Design review of the part built by this model. Coordinates are the model's own, in mm. Face numbers are marked on the shaded views. Round coordinates to 2 decimals unless told otherwise and drop trailing zeros. Order: outer loops, then holes, each group sorted by start corner. A loop starts at its lowest first (then second) coordinate and runs counter-clockwise, first axis right, second up. Notation, with made-up numbers: (14.5, 18.25) - (25.5, 18.25) arc R34 cw to (25.5, 49.25) - close; hole circle Ø6 at (51.5, 40.5). An arc over 180 degrees is marked (long way). Write item = value, one per line.
from build123d import *

# Parameters (mm, degrees)
SKETCH2_W           = 70
SKETCH2_H           = 50
BOSS_EXTRUDE1_DEPTH = 10
SKETCH3_R           = 4
CUT_EXTRUDE1_DEPTH  = 11
SKETCH5_R           = 8.5
CUT_EXTRUDE3_DEPTH  = 11


with BuildPart() as part:
    # Sketch2 → Boss-Extrude1 (new body)
    with BuildSketch(Plane(origin=(0, 0, 0), x_dir=(1, 0, 0), z_dir=(0, 1, 0))):
        Rectangle(SKETCH2_W, SKETCH2_H)
    extrude(amount=BOSS_EXTRUDE1_DEPTH)

    # Sketch3 → Cut-Extrude1 (cut, through all)
    with BuildSketch(Plane.XZ):
        with Locations((-25, 15)):
            Circle(SKETCH3_R)
        with Locations((25, 15)):
            Circle(SKETCH3_R)
    extrude(amount=-CUT_EXTRUDE1_DEPTH, mode=Mode.SUBTRACT)

    # Sketch5 → Cut-Extrude3 (cut, through all)
    with BuildSketch(Plane.XZ):
        with Locations((0, 4)):
            Circle(SKETCH5_R)
    extrude(amount=-CUT_EXTRUDE3_DEPTH, mode=Mode.SUBTRACT)


solid = part.part
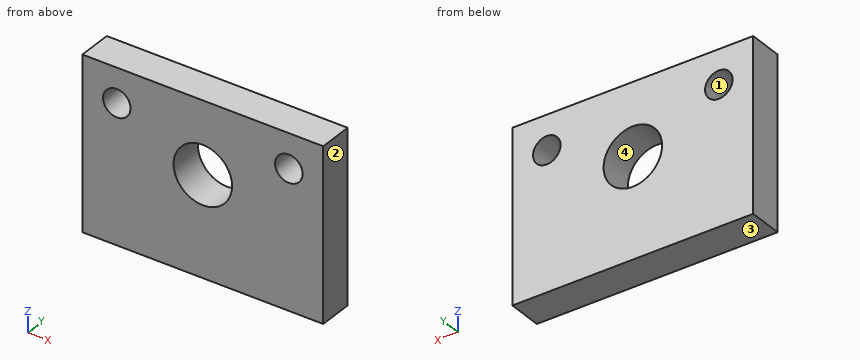
Item 1: The part is to be moulded in two halves that separate along Z. For the marked faces 1, 2, 3 and 4, say which applies: +Z half, -Z half, draft (parallel to the pull), parting line (faces both ways), or undercut.
Data:
face_1 = undercut
face_2 = draft
face_3 = -Z half
face_4 = undercut
Item 2: Take a section at A-A, the plane x = 25. State the section outline as (y, z) points.
Data:
outline = (0, -25) - (10, -25) - (10, 11) - (0, 11) - close; (0, 19) - (10, 19) - (10, 25) - (0, 25) - close
Item 3: Take a section at D-D, the plane z = 4. State the section outline as (x, y) points, and give its area (3 significant figures).
Data:
outline = (-35, 0) - (-8.5, 0) - (-8.5, 10) - (-35, 10) - close; (8.5, 0) - (35, 0) - (35, 10) - (8.5, 10) - close
area = 530 mm2
Item 4: Take a section at C-C, the plane z = 15. State the section outline as (x, y) points.
Data:
outline = (-35, 0) - (-29, 0) - (-29, 10) - (-35, 10) - close; (-21, 0) - (21, 0) - (21, 10) - (-21, 10) - close; (29, 0) - (35, 0) - (35, 10) - (29, 10) - close
Item 5: For line 1 along Z through (x, y) = (0, 5.5); line 2 along Z through (x, y) = (25, 4); line 3 along X through (y, z) = (9, -2.5), list the stretches that pass through material, from the lowest coordinate up. Write a range as [from, to].
Data:
line_1 = [-25, -4.5], [12.5, 25]
line_2 = [-25, 11], [19, 25]
line_3 = [-35, -5.48], [5.48, 35]
Item 6: Take a section at B-B, the plane y = 3. State the section outline as (x, z) points.
Data:
outline = (-35, -25) - (35, -25) - (35, 25) - (-35, 25) - close; hole circle Ø8 at (-25, 15); hole circle Ø17 at (0, 4); hole circle Ø8 at (25, 15)
